Autodesk Inventor part; units mm, degrees
ref_plane "YZ Plane" through (0, 0, 0) normal (1, 0, 0) x (0, 1, 0)
ref_plane "XZ Plane" through (0, 0, 0) normal (0, 1, 0) x (-1, 0, 0)
ref_plane "XY Plane" through (0, 0, 0) normal (0, 0, 1) x (1, 0, 0)
sketch "Sketch1" plane through (0, 0, 0) normal (0, 0, 1) x (1, 0, 0)
  line L0 (-16.019, 0) -> (-11.019, 0)
  line L1 (-16.019, 1.5) -> (-11.319, 1.5)
  line L2 (-16.019, 0) -> (-16.019, 2.85)
  line L3 (-17.669, 0) -> (-17.669, 1.425)
  line L4 (-11.019, 1.2) -> (-11.019, 0)
  line L5 (-16.369, 0) -> (-16.369, 2.85)
  line L6 (-16.019, 2.85) -> (-16.369, 2.85)
  arc A0 (-16.369, 2.85) -> (-17.669, 1.425) centre (-14.6489, -0.0247) ccw
  line L7 (-11.319, 1.5) -> (-11.019, 1.2)
  line L8 (-16.019, 0) -> (-17.669, 0)
  point P0 (0, 0)
  point P1 (-11.019, 1.5)
  dimension "d0" = 5
  dimension "d1" = 1.5
  dimension "d2" = 2.85
  dimension "d3" = 1.425
  dimension "d4" = 1.65
  dimension "d5" = 2.85
  dimension "d6" = 0.35
  dimension "d7" = 3.35
  dimension "d8" = 0.3
  dimension "d9" = 45
revolve "Revolution1" add sketch "Sketch1" angle 360 about axis through (-16.019, 0, 0) along (1, 0, 0)
sketch "Sketch2" plane through (-17.669, 0, 0) normal (-1, 0, 0) x (0, 0, 1)
  line L0 (-1, 0) -> (-0.5, 0.866)
  line L1 (-0.5, 0.866) -> (0.5, 0.866)
  line L2 (0.5, 0.866) -> (1, 0)
  line L3 (1, 0) -> (0.5, -0.866)
  line L4 (0.5, -0.866) -> (-0.5, -0.866)
  line L5 (-0.5, -0.866) -> (-1, 0)
  point P0 (0, 0)
  point P1 (0, 0)
  dimension "d11" = 2
extrude "Extrusion1" cut sketch "Sketch2" against normal blind 1
thread "Thread1"
properties part number "bolt_2_5mm" material "Steel, Mild, Welded"
Can you work these out from the model? Positions are in its coordinate system, mm. A direction names the side the tool comes from. Coordinates: 2 decimals unless noted, no trailing zeros. Write each loop counter-clockwise with the first axis right and the second up, starting at its lowest first coordinate (ties: lowest second). Pieces come first, ordered by that corner, then holes. Notation, with made-up numbers: (-4, 4) -> (11, 4) arc R4 cw to (11, 9) -> close; hole circle Ø1 at (86, -27). An arc over 180 degrees is marked (long way). Write each question's results on one line, items separated by ' | '. Start each with the question number.
Item 1: If we section it at A-A, the plane x = -14.25: Write out the boundary of the cut face in (y, z).
Item 2: I'm going to push flat-ended pins straight in: P1, Ø3, axis at x = -17, y = -2, coming from the +Z side; P2, Ø1, axis at x = -17, z = -1, coming from the +Y side; P3, Ø0.8, axis at x = -17, z = 0, coming from the -Y side. Where does each tip first touch, or does it pass through?
Item 3: Please list where these lines run through material, in increasing order: probe 1 along X at (y, z) = (0.15, 0.85); probe 2 along Y at (x, z) = (-17, 0.8); probe 3 along Z at (x, y) = (-17.5, 1.25).
Item 4: On a 3-axis mill with a long thin cutter (end or side, diameter ignored), from which of +Z, -Z, +X, -X, +Y, -Y can I reach the whole of each face in a straight line? I mean faces 1 (the cylindrical face through (-16.196, -2.262, 1.734)), 2 (the flat face through (-17.18, 0.43, -0.75)). Say none if no direction works.
Item 5: Thinking about a two-plate mould opening in Y: for faces 3 (the cylindrical face through (-13.64, -1.5, 0.07)), 4 (the flat face through (-16.019, 1.2, -1.2)), 5 (the flat face through (-16.669, 0, 0)), 6 (the flat face through (-17.18, -0.43, 0.75)), which applies, released by +Y, released by -Y, zero draft, split by the parting line, or undercut?
Answer block:
1) outline: circle Ø3 at (0, 0)
2) P1: z = 2.78 | P2: y = 2.62 | P3: y = -2.7
3) probe 1: -16.67 to -11.02 | probe 2: -2.22 to -0.35, 0.35 to 2.22 | probe 3: -1.2 to 1.2
4) face 1: +X, -X | face 2: -X
5) face 3: split by the parting line | face 4: zero draft | face 5: undercut | face 6: undercut
